The listing builds one solid part. Answer for the finished solid, in the listing's coordinates (mm). A direction names the side the tool comes from. Round coordinates to 2 decimals unless told otherwise and drop trailing zeros. Write each loop counter-clockwise with the first axis right and the second up, starting at its lowest first coordinate (ties: lowest second). Pieces come first, ordered by that corner, then holes.
from build123d import *

# Parameters (mm, degrees)
F0_W      = 25.4
F0_H      = 33.02
F2_DEPTH  = 19.05
F3_W      = 15.24
F3_H      = 13.97
F4_DEPTH  = 33.021
F5_W      = 2.54
F5_H      = 2.54
F6_DEPTH  = 33.021
F8_W      = 15.240135
F8_H      = 10.197046
F8_W_2    = 15.24
F8_H_2    = 10.16
F9_DEPTH  = 19.051
F11_R     = 5.715
F12_DEPTH = 152.4


with BuildPart() as f2:
    # F0 (on Front) → F2 (new body)
    with BuildSketch(Plane.XZ):
        with Locations((12.7, 16.51)):
            Rectangle(F0_W, F0_H)
    extrude(amount=-F2_DEPTH)

    # F3 (on face) → F4 (cut, through all)
    with BuildSketch(Plane.XY.offset(33.02)):
        with Locations((12.7, 6.985)):
            Rectangle(F3_W, F3_H)
    extrude(amount=-F4_DEPTH, mode=Mode.SUBTRACT)

    # F5 (on face) → F6 (cut, through all)
    with BuildSketch(Plane.XY.offset(33.02)):
        with Locations((3.81, 1.27)):
            Rectangle(F5_W, F5_H)
        with Locations((21.59, 1.27)):
            Rectangle(F5_W, F5_H)
    extrude(amount=-F6_DEPTH, mode=Mode.SUBTRACT)

    # F8 (on face) → F9 (cut, through all)
    with BuildSketch(Plane.XZ):
        with Locations((12.700067, 27.958523)):
            Rectangle(F8_W, F8_H)
        with Locations((12.7, 5.08)):
            Rectangle(F8_W_2, F8_H_2)
    extrude(amount=-F9_DEPTH, mode=Mode.SUBTRACT)

    # F11 (on face) → F12 (join)
    with BuildSketch(Plane(origin=(0, 19.05, 0), x_dir=(-1, 0, 0), z_dir=(0, 1, 0))):
        with Locations((-12.7, 16.51)):
            Circle(F11_R)
    extrude(amount=F12_DEPTH)


solid = f2.part
1. Straight lines are drawn through the part: line 1 along X through (y, z) = (122, 17); line 2 along Y through (x, z) = (4, 10); line 3 along Y through (x, z) = (15.5, 12.5). For each, find the intervals that lie inside material, in ascending order.
Geometry says:
line 1: x = 7.01 to 18.39
line 2: y = 2.54 to 19.05
line 3: y = 13.97 to 171.45
2. Given pin 1 (6 mm diameter, centred on x = 11.5, y = 52, fed in from +Z) (3 decimals); pin 2 (5 mm diameter, centred on x = 22.5, z = 25, fed in from +Y); pin 3 (4 mm diameter, centred on x = 17.5, y = 85, fed in from -Z), each flat-ended and moving along its own axis, determine where each tip first touches the part or whether it passes through.
Geometry says:
pin 1: stops at z = 22.225
pin 2: stops at y = 19.05
pin 3: stops at z = 11.53
3. Section D-D on z = 16.51 is taken. Determine the outline of the cut face in (x, y) (3 decimals).
Geometry says:
outline: (0, 0) - (2.54, 0) - (2.54, 2.54) - (5.08, 2.54) - (5.08, 13.97) - (20.32, 13.97) - (20.32, 2.54) - (22.86, 2.54) - (22.86, 0) - (25.4, 0) - (25.4, 19.05) - (18.415, 19.05) - (18.415, 171.45) - (6.985, 171.45) - (6.985, 19.05) - (0, 19.05) - close
4. Section C-C on x = 12.7 is taken. Determine the outline of the cut face in (y, z) (3 decimals).
Geometry says:
outline: (13.97, 10.16) - (19.05, 10.16) - (19.05, 10.795) - (171.45, 10.795) - (171.45, 22.225) - (19.05, 22.225) - (19.05, 22.86) - (13.97, 22.86) - close
5. Section B-B on z = 30 is taken. Determine the outline of the cut face in (x, y).
Geometry says:
outline: (0, 0) - (2.54, 0) - (2.54, 2.54) - (5.08, 2.54) - (5.08, 19.05) - (0, 19.05) - close; (20.32, 2.54) - (22.86, 2.54) - (22.86, 0) - (25.4, 0) - (25.4, 19.05) - (20.32, 19.05) - close
6. A tool of negligible diameter and unlimited length cuts with its end or side. For faces 1 (the face through (13, 16, 10.16)), 2 (the face through (20.32, 9, 11)), 3 (the face through (10.06, 94.18, 11.44)), 4 (the face through (20.32, 11, 28)), 5 (the face through (13, 13.97, 17)), from which of +Z, -Z, +X, -X, +Y, -Y can it reach the whole face along a straight path? Write none if from no direction.
Geometry says:
face 1: -Z, +Y, -Y
face 2: -Z, -Y
face 3: +Y
face 4: +Z, +Y, -Y
face 5: +Z, -Z, -Y
